from build123d import *

# Parameters (mm, degrees)
SKETCH1_W                 = 46
SKETCH1_H                 = 40.2
BOSS_EXTRUDE1_DEPTH       = 65.1
SKETCH3_R                 = 14
BOSS_EXTRUDE2_DEPTH       = 3
SKETCH4_R                 = 4.9
BOSS_EXTRUDE3_DEPTH       = 4.8
SKETCH7_W                 = 40.2
SKETCH7_H                 = 35.4
BOSS_EXTRUDE6_DEPTH       = 1
CHAMFER1_SIZE             = 6
CHAMFER1_SIZE2            = 5.1
MIRROR3_START             = 44.200099823
MIRROR3_OUTLINE_W         = 50
MIRROR3_OUTLINE_H         = 11
MIRROR3_DEPTH             = 3.885890521
CHAMFER1_OF_MIRROR8_SIZE2 = 5.1
CHAMFER1_OF_MIRROR8_SIZE  = 6
BOSS_EXTRUDE7_DEPTH       = 4.7625
SKETCH9_W                 = 40.2
SKETCH9_H                 = 61.1
BOSS_EXTRUDE8_DEPTH       = 41
SKETCH10_W                = 38
SKETCH10_H                = 38
BOSS_EXTRUDE9_DEPTH       = 9.3
SKETCH11_R                = 14
BOSS_EXTRUDE10_DEPTH      = 3
SKETCH12_R                = 4.9
BOSS_EXTRUDE11_DEPTH      = 4.8
BOSS_EXTRUDE12_REACH      = 145.093
SKETCH13_W                = 57.525
SKETCH13_H                = 40.156919592


# Read off the part's stored shape, not the designer's step: Mirror3
with BuildPart() as part:
    # Sketch1 → Boss-Extrude1 (new body)
    with BuildSketch(Plane(origin=(0, -14.5, 0), x_dir=(-1, 0, 0), z_dir=(0, 1, 0))):
        Rectangle(SKETCH1_W, SKETCH1_H)
    extrude(amount=BOSS_EXTRUDE1_DEPTH)

    # Sketch3 → Boss-Extrude2 (add)
    with BuildSketch(Plane.ZY.offset(-23)):
        Circle(SKETCH3_R)
    extrude(amount=-BOSS_EXTRUDE2_DEPTH)

    # Sketch4 → Boss-Extrude3 (add)
    with BuildSketch(Plane(origin=(26, 0, 0), x_dir=(0, 0, -1), z_dir=(1, 0, 0))):
        with Locations(Location((0, 0, 0), (0, 0, 180))):
            Circle(SKETCH4_R)
    extrude(amount=BOSS_EXTRUDE3_DEPTH)

    # Sketch7 → Boss-Extrude6 (add)
    with BuildSketch(Plane.ZY.offset(23)):
        with Locations((0, 32.9)):
            Rectangle(SKETCH7_W, SKETCH7_H)
    boss_extrude6 = extrude(amount=BOSS_EXTRUDE6_DEPTH)

    # Mirror1: Boss-Extrude6 across plane
    add(boss_extrude6.mirror(Plane(origin=(0, 0, 0), x_dir=(0, 0, 1), z_dir=(1, 0, 0))))

    # Chamfer1
    chamfer1_edges = [part.edges().sort_by_distance(p)[0] for p in [
        (0, 50.6, 20.1),
    ]]
    chamfer1_side = [part.faces().sort_by_distance(p)[0] for p in [
        (0, 18.392982971, 20.1),
    ]]
    chamfer(chamfer1_edges, length=CHAMFER1_SIZE, length2=CHAMFER1_SIZE2, reference=chamfer1_side[0])

    # Mirror3 outline → Mirror3 (cut)
    with BuildSketch(Plane(origin=(0, 0, 0), x_dir=(1, 0, 0), z_dir=(0, 0.6476484200955404, -0.7619393177594594)).offset(MIRROR3_START)):
        with Locations((0, -24.5)):
            Rectangle(MIRROR3_OUTLINE_W, MIRROR3_OUTLINE_H)
    mirror3 = extrude(amount=MIRROR3_DEPTH, mode=Mode.SUBTRACT)

    # Mirror8: Mirror3 across plane
    add(mirror3.mirror(Plane.ZX.offset(18.05)), mode=Mode.SUBTRACT)

    # Chamfer1 of Mirror8
    chamfer1_of_mirror8_edges = [part.edges().sort_by_distance(p)[0] for p in [
        (0, -14.5, 20.1),
    ]]
    chamfer(chamfer1_of_mirror8_edges, length=CHAMFER1_OF_MIRROR8_SIZE, length2=CHAMFER1_OF_MIRROR8_SIZE2)

    # Sketch8 → Boss-Extrude7 (add)
    with BuildSketch(Plane(origin=(24, 0, 0), x_dir=(0, 0, -1), z_dir=(1, 0, 0))):
        Polygon((20.1, 15.2), (8.9, 15.2), (-20.1, 31.2), (-20.1, 115.2), (8.9, 115.2), (8.9, 57.776470588), (20.1, 44.6), align=None)
    boss_extrude7 = extrude(amount=BOSS_EXTRUDE7_DEPTH)

    # Mirror4: Boss-Extrude7 across plane
    add(boss_extrude7.mirror(Plane(origin=(0, 0, 0), x_dir=(0, 0, 1), z_dir=(1, 0, 0))))



with BuildPart() as body_2:
    # Sketch9 → Boss-Extrude8 (new body)
    with BuildSketch(Plane(origin=(0, 116.7, 0), x_dir=(-1, 0, 0), z_dir=(0, 1, 0))):
        with Locations((0, -17.55)):
            Rectangle(SKETCH9_W, SKETCH9_H)
    extrude(amount=-BOSS_EXTRUDE8_DEPTH)


with BuildPart() as part_1:
    add(part.part)

    add(body_2.part)  # Boss-Extrude9 merges body 2
    # Sketch10 → Boss-Extrude9 (add)
    with BuildSketch(Plane.ZY.offset(-24)):
        with Locations((1.1, 96.2)):
            Rectangle(SKETCH10_W, SKETCH10_H)
    boss_extrude9 = extrude(amount=BOSS_EXTRUDE9_DEPTH)

    # Mirror6: Boss-Extrude9 across plane
    add(boss_extrude9.mirror(Plane(origin=(0, 0, 0), x_dir=(0, 0, 1), z_dir=(1, 0, 0))))

    # Sketch11 → Boss-Extrude10 (add)
    with BuildSketch(Plane(origin=(0, 116.7, 0), x_dir=(-1, 0, 0), z_dir=(0, 1, 0))):
        with Locations(Location((0, 0, 0), (0, 0, 68.213210702))):
            Circle(SKETCH11_R)
    extrude(amount=BOSS_EXTRUDE10_DEPTH)

    # Sketch12 → Boss-Extrude11 (add)
    with BuildSketch(Plane(origin=(0, 119.7, 0), x_dir=(1, 0, 0), z_dir=(0, 1, 0))):
        with Locations(Location((0, 0, 0), (0, 0, 270))):
            Circle(SKETCH12_R)
    extrude(amount=BOSS_EXTRUDE11_DEPTH)

    # Boss-Extrude12: up to this face of the body (flat: up to its plane)
    boss_extrude12_end = Plane(part_1.part.faces().sort_by_distance((0, -14.5, 0))[0])
    # Sketch13 → Boss-Extrude12 (add, up to the picked face)
    with BuildSketch(Plane(origin=(0, 116.7, 0), x_dir=(1, 0, 0), z_dir=(0, 1, 0)), mode=Mode.PRIVATE) as boss_extrude12_sk1:
        with Locations((0, -0.021540204)):
            Rectangle(SKETCH13_W, SKETCH13_H)
    boss_extrude12_tool1 = split(extrude(boss_extrude12_sk1.sketch, amount=-BOSS_EXTRUDE12_REACH, mode=Mode.PRIVATE), bisect_by=boss_extrude12_end, keep=Keep.BOTH, mode=Mode.PRIVATE)
    add(boss_extrude12_tool1.solids().sort_by(Axis((0, 116.7, 0.02154), (0, -1, 0)))[0])


solid = part_1.part
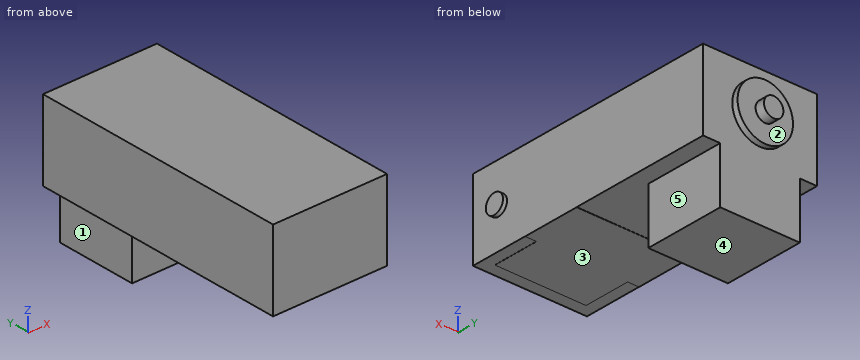
Design review of the part built by this model. Coordinates are the model's own, in mm. Face numbers are marked on the shaded views. A direction names the side the tool comes from. Round coordinates to 2 decimals unless told otherwise and drop trailing zeros. Loops run counter-clockwise (first coordinate to the right, second up) from the corner with the lowest first, then second, coordinate; pieces in that order, holes last. Notation, with made-up numbers: M -2.5,72.5 L 20.5,72.5 A17 ccw 20.5,100.5 Z; hole C -38,-1 d9. An arc over 180 degrees is marked long. Answer as a JSON object with one key per item and string values.
Item 1: We need section C-C on z = 0. Give the boundary of the cut face in (x, y), and give its area (3 significant figures).
Answer sheet:
{"outline": "M -28.76,-14.5 L 28.76,-14.5 L 28.76,-4.9 L 30.8,-4.9 L 30.8,4.9 L 28.76,4.9 L 28.76,116.7 L 14,116.7 L 14,119.7 L 4.9,119.7 L 4.9,124.5 L -4.9,124.5 L -4.9,119.7 L -14,119.7 L -14,116.7 L -28.76,116.7 Z", "area": "7,700 mm^2"}
Item 2: Machinability: for the marked faces 1, 2, 3, 4 and 5, which of the approach directions +Z, -Z, +X, -X, +Y, -Y give a long, thin tool a straight path to every point of the face, cutting with its end or side? Answer none if there is none.
Answer sheet:
{"face 1": "-Z, -X, +Y, -Y", "face 2": "+Y", "face 3": "-Z, +X, -X, -Y", "face 4": "-Z, +X, -X, +Y, -Y", "face 5": "-Z, +X, +Y, -Y"}
Item 3: Clearance check with flat-ended pins moving along their axes: P1, Ø1.5, axis at x = -15, z = -31.5, coming from the -Y side; P2, Ø16, axis at x = -9, y = 18, coming from the -Z side; P3, Ø5, axis at x = 2.5, z = 13.5, coming from the +Y side; P4, Ø22.5, axis at x = 9.5, z = -29, coming from the -Y side. State where each tip first meets the part, or that it passes through.
Answer sheet:
{"P1": "stops at y = 75.7", "P2": "stops at z = -20.1", "P3": "stops at y = 119.7", "P4": "stops at y = -14.5"}
Item 4: We need section B-B on x = 0. Give the boundary of the cut face in (y, z).
Answer sheet:
{"outline": "M -14.5,-20.06 L -8.55,-20.06 L -8.5,-20.1 L 44.6,-20.1 L 44.65,-20.06 L 75.7,-20.06 L 75.7,-48.1 L 116.7,-48.1 L 116.7,-14 L 119.7,-14 L 119.7,-4.9 L 124.5,-4.9 L 124.5,4.9 L 119.7,4.9 L 119.7,14 L 116.7,14 L 116.7,20.1 L -14.5,20.1 Z"}
Item 5: We need section A-A on y = 8. Give the boundary of the cut face in (x, z).
Answer sheet:
{"outline": "M -28.76,-20.06 L -23,-20.06 L -23,-20.1 L 23,-20.1 L 23,-20.06 L 28.76,-20.06 L 28.76,20.1 L -28.76,20.1 Z"}
Item 6: We need section D-D on y = 79.5. Give the boundary of the cut face in (x, z), and give its area (3 significant figures).
Answer sheet:
{"outline": "M -28.76,-20.06 L -20.1,-20.06 L -20.1,-48.1 L 20.1,-48.1 L 20.1,-20.06 L 28.76,-20.06 L 28.76,20.1 L -28.76,20.1 Z", "area": "3,440 mm^2"}
Item 7: Wall thickness on L1, parallel to Z at x = 24.5, y = 106.5; L2, parallel to Y at x = -5, z = -11; L3, parallel to Y at x = -11, z = -34: over which ranges is each line inside the solid? List them lowest first. Write a range as from..to.
Answer sheet:
{"L1": "z = -20.06..20.1", "L2": "y = -14.5..119.7", "L3": "y = 75.7..116.7"}
